```python
from build123d import *

# Parameters (mm, degrees)
SKETCH1_R                = 8
SKETCH1_R_2              = 3.5
BOSS_EXTRUDE1_DEPTH      = 3
SKETCH2_R                = 8
SKETCH2_R_2              = 5
BOSS_EXTRUDE2_DEPTH      = 6
WRAP3_SECTION_W          = 4
WRAP3_SECTION_H          = 2
WRAP3_ANGLE              = 57.295779513
WRAP3_SECTOR_2_SECTION_W = 4
WRAP3_SECTOR_2_SECTION_H = 2
WRAP3_SECTOR_2_ANGLE     = 57.295779513
CUT_EXTRUDE1_DEPTH       = 4
BOSS_EXTRUDE3_DEPTH      = 9


with BuildPart() as part:
    # Sketch1 → Boss-Extrude1 (new body)
    with BuildSketch(Plane.XY):
        Circle(SKETCH1_R)
        Circle(SKETCH1_R_2, mode=Mode.SUBTRACT)
    extrude(amount=BOSS_EXTRUDE1_DEPTH)

    # Sketch2 → Boss-Extrude2 (add)
    with BuildSketch(Plane.XY.offset(3)):
        Circle(SKETCH2_R)
        Circle(SKETCH2_R_2, mode=Mode.SUBTRACT)
    extrude(amount=BOSS_EXTRUDE2_DEPTH)

    # Wrap3 section (on wrap section) → Wrap3 (revolve, cut)
    with BuildSketch(Plane(origin=(0, 0, 0), x_dir=(-0.8779640629990781, -0.4787265441587198, 0), z_dir=(0.4787265441587198, -0.8779640629990781, 0))):
        with Locations((6, -8)):
            Rectangle(WRAP3_SECTION_W, WRAP3_SECTION_H)
    revolve(axis=Axis((0, 0, 0), (0, 0, -1)), revolution_arc=WRAP3_ANGLE, mode=Mode.SUBTRACT)

    # Wrap3 sector 2 section (on wrap section) → Wrap3 sector 2 (revolve, cut)
    with BuildSketch(Plane(origin=(0, 0, 0), x_dir=(0.8772005042746819, 0.4801242290285337, 0), z_dir=(-0.4801242290285337, 0.8772005042746819, 0))):
        with Locations((6, -8)):
            Rectangle(WRAP3_SECTOR_2_SECTION_W, WRAP3_SECTOR_2_SECTION_H)
    revolve(axis=Axis((0, 0, 0), (0, 0, -1)), revolution_arc=WRAP3_SECTOR_2_ANGLE, mode=Mode.SUBTRACT)

    # Sketch5 → Cut-Extrude1 (cut)
    with BuildSketch(Plane(origin=(0, 0, 0), x_dir=(-1, 0, 0), z_dir=(0, 0, -1))):
        with BuildLine():
            Line((-1.1, 6.710439628), (-1.1, 7.924014134))
            ThreePointArc((-1.1, 7.924014134), (0, -8), (1.1, 7.924014134))
            Line((1.1, 7.924014134), (1.1, 6.710439628))
            ThreePointArc((1.1, 6.710439628), (0, -6.8), (-1.1, 6.710439628))
        make_face()
    extrude(amount=-CUT_EXTRUDE1_DEPTH, mode=Mode.SUBTRACT)

    # Sketch6 → Boss-Extrude3 (add)
    with BuildSketch(Plane(origin=(0, 0, 0), x_dir=(-1, 0, 0), z_dir=(0, 0, -1))):
        with BuildLine():
            Line((-1.1, 7.731159285), (-1.1, 8.310439628))
            Line((-1.1, 8.310439628), (1.1, 8.310439628))
            Line((1.1, 8.310439628), (1.1, 7.731159285))
            ThreePointArc((1.1, 7.731159285), (0, 7.807145151), (-1.1, 7.731159285))
        make_face()
    extrude(amount=-BOSS_EXTRUDE3_DEPTH)


solid = part.part
```
Work out the finished part from the listing and answer in its coordinate system (mm). A direction names the side the tool comes from. Round coordinates to 2 decimals unless told otherwise and drop trailing zeros. Write each loop counter-clockwise with the first axis right and the second up, starting at its lowest first coordinate (ties: lowest second). Pieces come first, ordered by that corner, then holes. Notation, with made-up numbers: (89, 14.5) - (107, 14.5) arc R30 cw to (107, 52.5) - close; hole circle Ø8 at (82, 31.25). An arc over 180 degrees is marked (long way). Return JSON: item names as keys, results as strings. Group by question number.
Q1. The part is cut by section A-A on x = 0. Write down the section's boundary in (y, z).
Q2. For faces 1 (the flat face through (2.2, -3.3, 3)), 2 (the flat face through (-5.688, -3.102, 7.986)), 3 (the flat face through (6, -4, 4)), 4 (the flat face through (5.688, -3.102, 7.986)), determine the directions among +Z, -Z, +X, -X, +Y, -Y from which every point of the face is accessible in a straight line to the end or side of a thin tool.
Q3. The part is cut by section C-C on z = 3.5. Write down the section's boundary in (x, y), then the cut area to 3 significant figures.
Q4. The part is cut by section B-B on y = 0. Write down the section's boundary in (x, z), then the cut area to 3 significant figures.
Q5. The part is cut by section D-D on x = -2.75. Write down the section's boundary in (y, z), then the cut area to 3 significant figures.
Q6. Find the intervals of material crossed by L1, parallel to X at y = 0, z = 5.05; L2, parallel to Y at x = 0, z = 0.7; L3, parallel to Y at x = 0, z = 4.8, in increasing order.
Q7. Each of these flat-tipped pins is pushed along its axis until it touches: pin 1 Ø9 at (x, y) = (0, 0) entering from +Z; pin 2 Ø4 at (x, y) = (-6, 0) entering from +Z; pin 3 Ø2 at (y, z) = (-2.5, 2) entering from -X. Where does it stop, or does it pass through?
Q8. The mould has two halves that part along Y. Classify faces 5 (the flat face through (1.1, 8, 2)), 6 (the flat face through (-6, 0, 7)), 7 (the cylindrical face through (0, -8, 6)), 8 (the flat face through (6, 0, 7)): released by +Y, released by -Y, zero draft, split by the parting line, or undercut.
Solved:
{
 "1": {"outline": "(-8, 4) - (-6.8, 4) - (-6.8, 0) - (-3.5, 0) - (-3.5, 3) - (-5, 3) - (-5, 9) - (-8, 9) - close; (3.5, 0) - (8.31, 0) - (8.31, 9) - (5, 9) - (5, 3) - (3.5, 3) - close"},
 "2": {"face 1": "+Z", "face 2": "+Z, -X", "face 3": "-Z", "face 4": "+Z, +X"},
 "3": {"outline": "(-1.1, 6.71) arc R6.8 ccw (long way) to (1.1, 6.71) - (1.1, 8.31) - (-1.1, 8.31) - close; hole circle Ø10 at (0, 0)", "area": "70.1 mm²"},
 "4": {"outline": "(-8, 4) - (-6.8, 4) - (-6.8, 0) - (-3.5, 0) - (-3.5, 3) - (-5, 3) - (-5, 7) - (-8, 7) - close; (3.5, 0) - (6.8, 0) - (6.8, 4) - (8, 4) - (8, 7) - (5, 7) - (5, 3) - (3.5, 3) - close", "area": "41.4 mm²"},
 "5": {"outline": "(-7.51, 4) - (-6.22, 4) - (-6.22, 0) - (-2.17, 0) - (-2.17, 3) - (-4.18, 3) - (-4.18, 9) - (-7.51, 9) - close; (2.17, 0) - (6.22, 0) - (6.22, 4) - (7.51, 4) - (7.51, 9) - (4.18, 9) - (4.18, 3) - (2.17, 3) - close", "area": "61.8 mm²"},
 "6": {"L1": "-8 to -5, 5 to 8", "L2": "-6.8 to -3.5, 3.5 to 8.31", "L3": "-8 to -5, 5 to 8.31"},
 "7": {"pin 1": "z = 3", "pin 2": "z = 7", "pin 3": "x = -6.63"},
 "8": {"face 5": "zero draft", "face 6": "undercut", "face 7": "split by the parting line", "face 8": "undercut"}
}
